The model under review builds one solid part; all positions refer to its coordinate system, in mm. Face numbers are marked on the shaded views. A direction names the side the tool comes from. Round coordinates to 2 decimals unless told otherwise and drop trailing zeros. Write each loop counter-clockwise with the first axis right and the second up, starting at its lowest first coordinate (ties: lowest second). Pieces come first, ordered by that corner, then holes. Notation, with made-up numbers: M -38,2 L -13,2 A18 cw -13,20 Z; hole C 18,43.25 d5. An arc over 180 degrees is marked long. One line per item, written item: value. Start each with the question number.
1) Wall thickness on probe 1 along Y at (x, z) = (115, -15); probe 2 along Z at (x, y) = (88, 14.5); probe 3 along Z at (x, y) = (24, 10): over which ranges is each line inside the solid? List them lowest first.
2) Take a section at A-A, the plane z = -9. Write out the cut boundary in (x, y).
3) Take a section at D-D, the plane x = 12. Write out the cut boundary in (y, z) (1 decimal), and give its area (3 significant figures).
4) For P1, Ø0.5, axis at x = 9.5, y = 1, coming from the +Z side (3 decimals), flat-tipped, find the tip position at first contact; note if it passes through.
5) Take a section at C-C, the plane x = 96. Write out the cut boundary in (y, z), and give its area (3 significant figures).
6) Tool access review of the marked faces 1 and 2: name each direction out of +Z, -Z, +X, -X, +Y, -Y from which nothing blocks a thin tool from reaching the whole face with its end or side.
7) Take a section at B-B, the plane y = 13. Write out the cut boundary in (x, z), and give its area (3 significant figures).
8) Mouldability with a two-part tool opening along Y and no side actions: class the marked faces 3, 4, 5 and 6 as +Y half, -Y half, draft (parallel to the pull), parting line (faces both ways), or undercut.
Autodesk Inventor part; units mm, degrees
ref_plane "YZ Plane" through (0, 0, 0) normal (1, 0, 0) x (0, 1, 0)
ref_plane "XZ Plane" through (0, 0, 0) normal (0, 1, 0) x (-1, 0, 0)
ref_plane "XY Plane" through (0, 0, 0) normal (0, 0, 1) x (1, 0, 0)
sketch "Sketch1" plane through (0, 0, 0) normal (1, 0, 0) x (0, 1, 0)
  line L0 (0, 0) -> (25.4, 0)
  line L1 (25.4, 0) -> (25.4, -50.8)
  line L2 (25.4, -50.8) -> (0, -50.8)
  line L3 (0, -50.8) -> (0, 0)
  line L4 (23.8125, -1.5875) -> (1.5875, -1.5875)
  line L5 (1.5875, -1.5875) -> (1.5875, -49.2125)
  line L6 (1.5875, -49.2125) -> (23.8125, -49.2125)
  line L7 (23.8125, -49.2125) -> (23.8125, -1.5875)
  dimension "d0" = 25.4
  dimension "d1" = 50.8
  dimension "d2" = 1.5875
extrude "Extrusion1" add sketch "Sketch1" along normal blind 133.35
sketch "Sketch2" plane through (0, 25.4, 0) normal (0, 1, 0) x (1, 0, 0)
  line L0 (0, 0) -> (25.4, 0)
  line L1 (25.4, 0) -> (25.4, 15.875)
  line L2 (25.4, 15.875) -> (0, 15.875)
  line L3 (0, 15.875) -> (0, 0)
  dimension "d5" = 25.4
  dimension "d6" = 15.875
extrude "Extrusion2" cut sketch "Sketch2" against normal blind 82.55
properties part number "FRA_SideUpperSupport_003" material "Aluminum 6061"
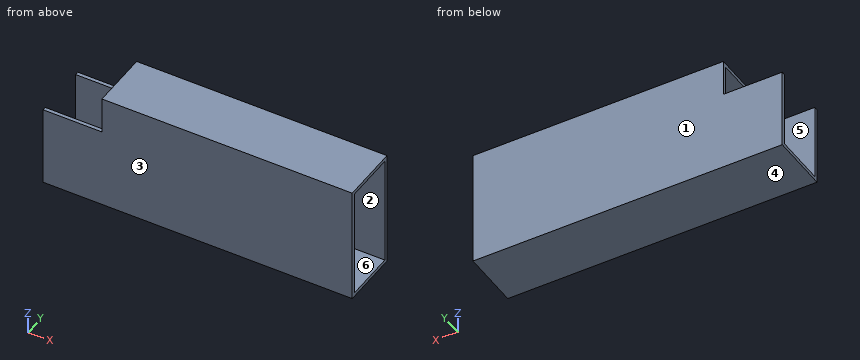
Checked values:
1. probe 1: y = 0 to 1.59, 23.81 to 25.4
1. probe 2: z = -50.8 to -49.21, -1.59 to 0
1. probe 3: z = -50.8 to -49.21
2. outline: M 25.4,0 L 133.35,0 L 133.35,1.59 L 25.4,1.59 Z; M 25.4,23.81 L 133.35,23.81 L 133.35,25.4 L 25.4,25.4 Z
3. outline: M 0,-50.8 L 25.4,-50.8 L 25.4,-15.9 L 23.8,-15.9 L 23.8,-49.2 L 1.6,-49.2 L 1.6,-15.9 L 0,-15.9 Z
3. area: 146 mm2
4. P1: stops at z = -15.875
5. outline: M 0,-50.8 L 25.4,-50.8 L 25.4,0 L 0,0 Z; hole M 1.59,-49.21 L 23.81,-49.21 L 23.81,-1.59 L 1.59,-1.59 Z
5. area: 232 mm2
6. face 1: +Z, -Z, +X, -X, +Y
6. face 2: +X, -X
7. outline: M 0,-50.8 L 133.35,-50.8 L 133.35,-49.21 L 0,-49.21 Z; M 25.4,-1.59 L 133.35,-1.59 L 133.35,0 L 25.4,0 Z
7. area: 383 mm2
8. face 3: -Y half
8. face 4: draft
8. face 5: undercut
8. face 6: undercut
